Drawing for the job (mm, zero at the part's lowest x, y, z). A direction names the side the tool comes from. Give positions to 0.01 mm unless a question says otherwise; leave off trailing zeros. Loops run counter-clockwise (first coordinate to the right, second up) from the corner with the lowest first, then second, coordinate; pieces in that order, holes last. Notation, with made-up numbers: (-22, 71.25) -> (24, 71.25) arc R17 cw to (24, 75.25) -> close; hole circle Ø8 at (66.25, 14). An arc over 180 degrees is marked (long way). Use CSV: the item, a comma, the result in double quotes. Start each with the question number.
(1) Cut at A-A on y = 7.5. Write the cut outline in (x, z), then the cut area to 3 significant figures.
(2) 3-axis set-ups, long thin cutter, end or side, ignore diameter. For the marked faces 1, 2 and 3: which of +Z, -Z, +X, -X, +Y, -Y reach the whole face in a straight line?
(3) Cut at D-D on z = 31. Write the cut outline in (x, y), then the cut area to 3 significant figures.
(4) Cut at B-B on z = 8. Write the cut outline in (x, y).
(5) Flat gauge pins, fed straight in: pin 1 (3 mm diameter, centred on x = 19.5, z = 26, fed in from -Y); pin 2 (7.5 mm diameter, centred on x = 20, y = 6.5, fed in from +Z); pin 3 (8 mm diameter, centred on x = 25.5, z = 15, fed in from -Y); pin 4 (5 mm diameter, centred on x = 20.5, z = 29, fed in from +Y). Where does each tip first touch, or does it go through?
(6) Drill centre lines: probe 1 along X at (y, z) = (10.5, 46); probe 2 along Z at (x, y) = (25, 22.5); probe 3 along Z at (x, y) = (4, 4.5). Where is each one in solid material? Low to high.
(7) Cut at C-C on y = 26. Write the cut outline in (x, z), then the cut area to 3 significant figures.
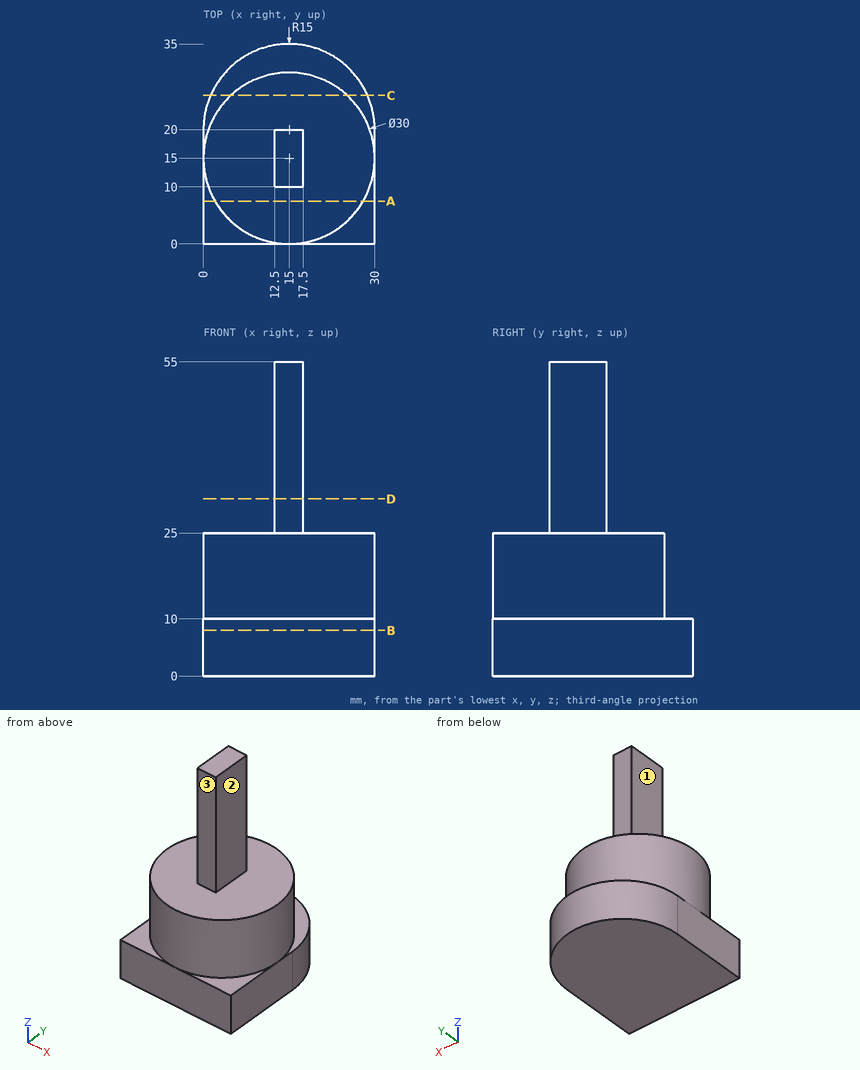
Check result:
1,outline,"(0, 0) -> (30, 0) -> (30, 10) -> (27.99, 10) -> (27.99, 25) -> (2.01, 25) -> (2.01, 10) -> (0, 10) -> close"
1,area,"690 mm²"
2,face 1,"+Z, -X, +Y, -Y"
2,face 2,"+Z, +X, +Y, -Y"
2,face 3,"+Z, +X, -X, -Y"
3,outline,"(12.5, 10) -> (17.5, 10) -> (17.5, 20) -> (12.5, 20) -> close"
3,area,"50.0 mm²"
4,outline,"(0, 0) -> (30, 0) -> (30, 20) arc R15 ccw to (0, 20) -> close"
5,pin 1,"y = 0.39"
5,pin 2,"z = 25"
5,pin 3,"y = 1.48"
5,pin 4,"through"
6,probe 1,"12.5 to 17.5"
6,probe 2,"0 to 25"
6,probe 3,"0 to 10"
7,outline,"(1.25, 0) -> (28.75, 0) -> (28.75, 10) -> (25.2, 10) -> (25.2, 25) -> (4.8, 25) -> (4.8, 10) -> (1.25, 10) -> close"
7,area,"581 mm²"
